Could you check a few things on this model? Use its own coordinates, in mm. A direction names the side the tool comes from. Coordinates: 2 decimals unless noted, no trailing zeros. Write each loop counter-clockwise with the first axis right and the second up, starting at its lowest first coordinate (ties: lowest second). Pieces come first, ordered by that corner, then holes. Notation, with made-up numbers: M 4.5,11 L 21.5,11 A16 ccw 21.5,23 Z; hole C 73.25,24.5 d1. An arc over 180 degrees is marked long. Write item = value, one per line.
```python
from build123d import *

# Parameters (mm, degrees)
F0_W      = 203.2
F0_H      = 203.2
F1_DEPTH  = 15.24
F2_R      = 9.525
F3_DEPTH  = 25.4
F4_R      = 6.35
F5_DEPTH  = 19.05
F6_R      = 9.525
F7_DEPTH  = 25.4
F8_R      = 6.35
F9_DEPTH  = 19.05
F10_W     = 66.012211
F10_H     = 227.670602
F11_DEPTH = 81.788
F12_W     = 0.028826
F12_H     = 5.976447
F13_DEPTH = 59.182


with BuildPart() as f1:
    # F0 (on Top) → F1 (new body)
    with BuildSketch(Plane.XY):
        Rectangle(F0_W, F0_H)
    extrude(amount=F1_DEPTH)

    # F2 (on face) → F3 (join)
    with BuildSketch(Plane.XY.offset(15.24)):
        Circle(F2_R)
        with Locations((62.23, 0)):
            Circle(F2_R)
        with Locations((-45.293553, 42.673961)):
            Circle(F2_R)
        with Locations((62.23, -62.23)):
            Circle(F2_R)
    extrude(amount=F3_DEPTH)

    # F4 (on face) → F5 (join)
    with BuildSketch(Plane.XY.offset(40.64)):
        with Locations((-45.293553, 42.673961)):
            Circle(F4_R)
        Circle(F4_R)
        with Locations((62.23, -62.23)):
            Circle(F4_R)
        with Locations((62.23, 0)):
            Circle(F4_R)
    extrude(amount=F5_DEPTH)

    # F6 (on face) → F7 (join)
    with BuildSketch(Plane.XY.offset(15.24)):
        with Locations((-42.088444, -45.838148)):
            Circle(F6_R)
    extrude(amount=F7_DEPTH)

    # F8 (on face) → F9 (join)
    with BuildSketch(Plane.XY.offset(40.64)):
        with Locations((-42.088444, -45.838148)):
            Circle(F8_R)
    extrude(amount=F9_DEPTH)

    # F10 (on face) → F11 (cut)
    with BuildSketch(Plane.XY.offset(59.69)):
        with Locations((81.731911, -7.860381)):
            Rectangle(F10_W, F10_H)
    extrude(amount=-F11_DEPTH, mode=Mode.SUBTRACT)

    # F12 (on face) → F13 (cut, symmetric)
    with BuildSketch(Plane.XY.offset(15.24)):
        Polygon((-15.059947, -28.248059), (-113.846987, -28.248059), (-113.846987, -116.091147), (57.950988, -116.091147), (57.950988, -28.248059), (-15.031121, -28.248059), (-15.031121, -34.224506), (-15.059947, -34.224506), align=None)
        with Locations((-15.045534, -31.236282)):
            Rectangle(F12_W, F12_H)
    extrude(amount=F13_DEPTH, both=True, mode=Mode.SUBTRACT)


solid = f1.part
```
Item 1: Imagine slicing it at D-D (y = 83.5). Write out the boundary of the cut face in (x, z).
Numbers:
outline = M -101.6,0 L 48.73,0 L 48.73,15.24 L -101.6,15.24 Z
Item 2: Imagine slicing it at B-B (x = 0). Write out the boundary of the cut face in (y, z) (3 decimals), and give its area (3 significant figures).
Numbers:
outline = M -28.248,0 L 101.6,0 L 101.6,15.24 L 9.525,15.24 L 9.525,40.64 L 6.35,40.64 L 6.35,59.69 L -6.35,59.69 L -6.35,40.64 L -9.525,40.64 L -9.525,15.24 L -28.248,15.24 Z
area = 2,700 mm²
Item 3: Imagine slicing it at A-A (y = 0). Write out the boundary of the cut face in (x, z) (3 decimals).
Numbers:
outline = M -101.6,0 L 48.726,0 L 48.726,15.24 L 9.525,15.24 L 9.525,40.64 L 6.35,40.64 L 6.35,59.69 L -6.35,59.69 L -6.35,40.64 L -9.525,40.64 L -9.525,15.24 L -101.6,15.24 Z
Item 4: Imagine slicing it at C-C (z = 33.5). Write out the boundary of the cut face in (x, y) (3 decimals).
Numbers:
outline = C -45.294,42.674 d19.05; C 0,0 d19.05
Item 5: For faces 1 (the face through (-101.6, 36, 8)), 2 (the face through (2, -6.2, 40.64)), which set-ups out of +Z, -Z, +X, -X, +Y, -Y let a thin tool reach every point of the face, with its end or its side?
Numbers:
face_1 = +Z, -Z, -X, +Y, -Y
face_2 = +Z
Item 6: If I drill on line 1 along Z through (x, y) = (-56.5, 47.5); line 2 along Y through (x, z) = (-45.5, 44); line 3 along Y through (x, z) = (3.5, 35.5), over which ranges is the centre line in solid material (lowest first)?
Numbers:
line_1 = 0 to 15.24
line_2 = 36.33 to 49.02
line_3 = -8.86 to 8.86
Item 7: I'm going to push flat-ended pins straight in: P1, Ø3, axis at x = -41, z = 25, coming from the -Y side; P2, Ø6, axis at x = 14.5, y = -1, coming from the +Z side; P3, Ø10, axis at x = -45, z = 41, coming from the +Y side. Where does each tip first touch, or does it pass through?
Numbers:
P1 = 33.57
P2 = 15.24
P3 = 52.2
